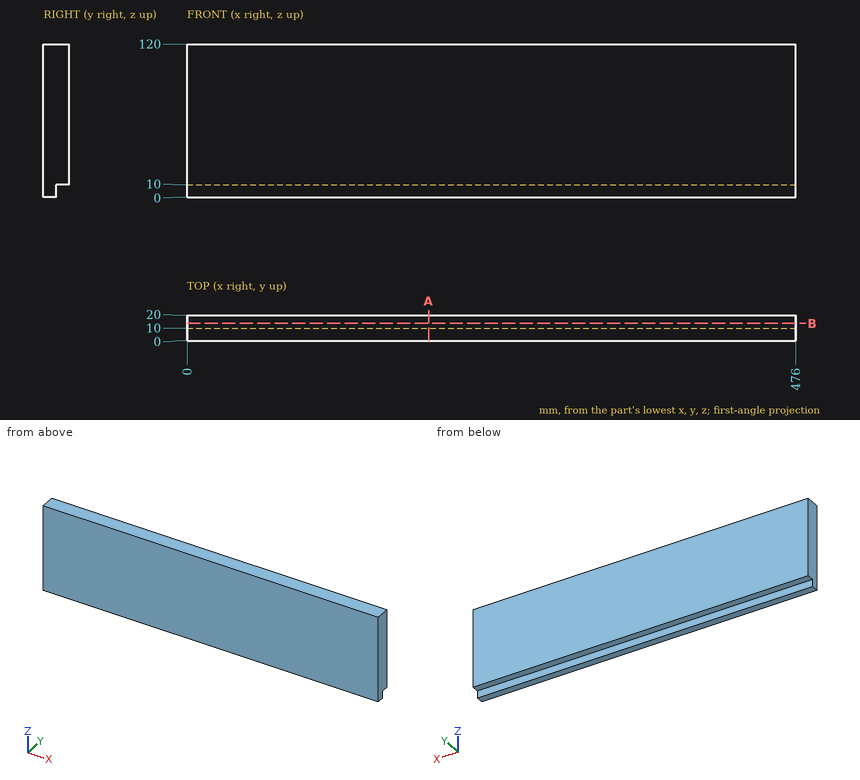
Print and shaded views of the part. All mm, measured from the part's lowest x, y and z. Coordinates: 2 decimals unless noted, no trailing zeros. Order: outer loops, then holes, each group sorted by start corner. A loop starts at its lowest first (then second) coordinate and runs counter-clockwise, first axis right, second up. Notation, with made-up numbers: (33.25, 53.5) -> (50.25, 53.5) arc R27 ccw to (50.25, 86.5) -> close; hole circle Ø9 at (-2, 82.25). An arc over 180 degrees is marked (long way). Answer as a JSON object with one key per item and string values. Group by question number.
1) Drill centre line: L1, parallel to Z at x = 70, y = 10.75. Where is it in solid material? Low to high.
2) Flat gauge pins, fed straight in: pin 1 (6 mm diameter, centred on y = 2, z = 86.5, fed in from -X); pin 2 (8 mm diameter, centred on x = 129, y = 15, fed in from -Z); pin 3 (3 mm diameter, centred on x = 169.5, z = 3.5, fed in from +Y). Where does each tip first touch, or does it go through?
3) Cut at A-A, the plane x = 189. Write the cut outline in (y, z).
4) Cut at B-B, the plane y = 13.75. Write the cut outline in (x, z), then the cut area to 3 significant figures.
Check values:
{
 "1": {"L1": "z = 10 to 120"},
 "2": {"pin 1": "stops at x = 0", "pin 2": "stops at z = 10", "pin 3": "stops at y = 10"},
 "3": {"outline": "(0, 0) -> (10, 0) -> (10, 10) -> (20, 10) -> (20, 120) -> (0, 120) -> close"},
 "4": {"outline": "(0, 10) -> (476, 10) -> (476, 120) -> (0, 120) -> close", "area": "52,400 mm²"}
}
